Model file for the job. Use its own axes, mm. A direction names the side the tool comes from. Coordinates: 2 decimals unless noted, no trailing zeros. Write each loop counter-clockwise with the first axis right and the second up, starting at its lowest first coordinate (ties: lowest second). Pieces come first, ordered by that corner, then holes. Notation, with made-up numbers: M 25.25,-27.75 L 58.25,-27.75 A22 ccw 58.25,4.25 Z; hole C -3,40 d5. An arc over 180 degrees is marked long. Use CSV: the item, a comma, the result in double quotes. Start each with the question number.
from build123d import *

# Parameters (mm, degrees)
SKETCH1_W                        = 70
SKETCH1_H                        = 100
SKETCH1_W_2                      = 58
SKETCH1_H_2                      = 88
MAIN_BODY_DEPTH                  = 50
BACK_WIRE_HOLE_REACH             = 102
SKETCH3_R                        = 1.5
FRONT_WIRE_HOLE_REACH            = 102
SKETCH6_R                        = 1.5
SKETCH4_W                        = 70
SKETCH4_H                        = 6
BACK_LIP_DEPTH                   = 10
SKETCH5_R                        = 1.5
BACK_LIP_HOLES_DEPTH             = 35
SKETCH2_R                        = 1.5
GEARED_ARM_HOLE_DEPTH            = 6
SKETCH10_W                       = 23
SKETCH10_H                       = 8.7393957
SERVO_MOUNT_MAIN_EXTRUSION_DEPTH = 58
WING_CONNECTION_SLOT_DEPTH       = 6


with BuildPart() as part:
    # Sketch1 → main_body (new body)
    with BuildSketch(Plane(origin=(0, 0, 0), x_dir=(1, 0, 0), z_dir=(0, 1, 0))):
        with Locations((0, -1.59009009)):
            Rectangle(SKETCH1_W, SKETCH1_H)
        with Locations((0, -1.59009009)):
            Rectangle(SKETCH1_W_2, SKETCH1_H_2, mode=Mode.SUBTRACT)
    extrude(amount=MAIN_BODY_DEPTH)

    # Sketch3 → back_wire_hole (cut, up to next)
    with BuildSketch(Plane.XY.offset(51.59009009), mode=Mode.PRIVATE) as back_wire_hole_sk1:
        with Locations((0, 25)):
            Circle(SKETCH3_R)
    back_wire_hole_tool1 = extrude(back_wire_hole_sk1.sketch, amount=-BACK_WIRE_HOLE_REACH, mode=Mode.PRIVATE) & part.part
    add(back_wire_hole_tool1.solids().sort_by_distance((0, 25, 51.59009))[0], mode=Mode.SUBTRACT)

    # Sketch6 → front_wire_hole (cut, up to next)
    with BuildSketch(Plane(origin=(0, 0, -48.40990991), x_dir=(-1, 0, 0), z_dir=(0, 0, -1)), mode=Mode.PRIVATE) as front_wire_hole_sk1:
        with Locations((0, 25)):
            Circle(SKETCH6_R)
    front_wire_hole_tool1 = extrude(front_wire_hole_sk1.sketch, amount=-FRONT_WIRE_HOLE_REACH, mode=Mode.PRIVATE) & part.part
    add(front_wire_hole_tool1.solids().sort_by_distance((0, 25, -48.40991))[0], mode=Mode.SUBTRACT)

    # Sketch4 → back_lip (add)
    with BuildSketch(Plane.XY.offset(51.59009009)):
        with Locations((0, 31)):
            Rectangle(SKETCH4_W, SKETCH4_H)
    back_lip = extrude(amount=BACK_LIP_DEPTH)

    # back_lip_mirror: back_lip across plane
    add(back_lip.mirror(Plane.ZX.offset(25)))

    # Sketch5 → back_lip_holes (cut, through all)
    with BuildSketch(Plane(origin=(0, 34, 0), x_dir=(1, 0, 0), z_dir=(0, 1, 0))):
        with Locations((4, -55.59009009)):
            Circle(SKETCH5_R)
        with Locations((30, -55.59009009)):
            Circle(SKETCH5_R)
        with Locations((-30, -55.59009009)):
            Circle(SKETCH5_R)
        with Locations((-4, -55.59009009)):
            Circle(SKETCH5_R)
    extrude(amount=-BACK_LIP_HOLES_DEPTH, mode=Mode.SUBTRACT)

    # Sketch2 → geared_arm_hole (cut)
    with BuildSketch(Plane(origin=(35, 0, 0), x_dir=(0, 0, -1), z_dir=(1, 0, 0))):
        with Locations((-1.59009009, 25)):
            Circle(SKETCH2_R)
    geared_arm_hole = extrude(amount=-GEARED_ARM_HOLE_DEPTH, mode=Mode.SUBTRACT)

    # geared_arm_hole_mirror: geared_arm_hole across plane
    add(geared_arm_hole.mirror(Plane(origin=(0, 0, 0), x_dir=(0, 0, 1), z_dir=(1, 0, 0))), mode=Mode.SUBTRACT)

    # Sketch10 → servo_mount_main_extrusion (add)
    with BuildSketch(Plane(origin=(-29, 0, 0), x_dir=(0, 0, -1), z_dir=(1, 0, 0))):
        with Locations((32.100688533, 4.36969785)):
            Rectangle(SKETCH10_W, SKETCH10_H)
        with Locations((32.100688533, 45.63030215)):
            Rectangle(SKETCH10_W, SKETCH10_H)
    extrude(amount=SERVO_MOUNT_MAIN_EXTRUSION_DEPTH)

    # Sketch11 → wing_connection_slot (cut)
    with BuildSketch(Plane(origin=(35, 0, 0), x_dir=(0, 0, -1), z_dir=(1, 0, 0))):
        with BuildLine():
            ThreePointArc((-32.317240778, 42.63125), (-33.09009009, 25), (-32.317240778, 7.36875))
            ThreePointArc((-32.317240778, 7.36875), (-30.691743999, 6.005753221), (-29.32874722, 7.63125))
            ThreePointArc((-29.32874722, 7.63125), (-30.09009009, 25), (-29.32874722, 42.36875))
            ThreePointArc((-29.32874722, 42.36875), (-30.691743999, 43.994246779), (-32.317240778, 42.63125))
        make_face()
    wing_connection_slot = extrude(amount=-WING_CONNECTION_SLOT_DEPTH, mode=Mode.SUBTRACT)

    # wing_connection_slot_mirror: wing_connection_slot across plane
    add(wing_connection_slot.mirror(Plane(origin=(0, 0, 0), x_dir=(0, 0, 1), z_dir=(1, 0, 0))), mode=Mode.SUBTRACT)


solid = part.part
1) Two-plate mould, pull along X, no slides. Class faces 1 (the face through (0, 8, 51.59)), 2 (the face through (28.89, 19.04, 54.58)), 3 (the face through (0, 4, -20.601)): pulls with the +X half, pulls with the -X half, needs draft (parallel to the pull), parting line crosses it, or undercut.
2) Band-saw the part on C-C on x = -14. List the corners of the cut face in (y, z), then the cut area to 3 significant figures.
3) Band-saw the part on A-A on x = 4. List the corners of the cut face in (y, z), then the cut area to 3 significant figures.
4) Tool access for faces 4 (the face through (0, 41.261, -31)), 5 (the face through (-32.04, 24.76, 30.09)), 6 (the face through (0, 42, 51.59)), 7 (the face through (0, 27, 51.59)): list every direction of +Z, -Z, +X, -X, +Y, -Y with a clear straight run to the whole face (end or side of a thin tool).
5) Drop flat-ended pins along their axis: P1, Ø13, axis at x = -14.5, y = 7, coming from the +Z side; P2, Ø11, axis at x = 5.5, z = 57.5, coming from the +Y side; P3, Ø5, axis at x = -8, z = 57, coming from the -Y side. Give the stop position or say it passes through.
6) Wall check: L1, parallel to Z at x = -12, y = 16.5; L2, parallel to X at y = 25, z = 28.5; L3, parallel to Y at x = 18, z = -33. Give the ranges that are in metal, low to high. Write a range as [from, to].
7) Band-saw the part on B-B on z = 15. List the corners of the cut face in (x, y).
8) Band-saw the part on D-D on z = -40. List the corners of the cut face in (x, y), then the cut area to 3 significant figures.
Findings below:
1,face 1,"needs draft"
1,face 2,"undercut"
1,face 3,"undercut"
2,outline,"M 0,-48.41 L 50,-48.41 L 50,-20.6 L 41.26,-20.6 L 41.26,-42.41 L 8.74,-42.41 L 8.74,-20.6 L 0,-20.6 Z; M 0,45.59 L 50,45.59 L 50,51.59 L 34,51.59 L 34,61.59 L 28,61.59 L 28,51.59 L 22,51.59 L 22,61.59 L 16,61.59 L 16,51.59 L 0,51.59 Z"
2,area,"1,100 mm2"
3,outline,"M 0,-48.41 L 50,-48.41 L 50,-20.6 L 41.26,-20.6 L 41.26,-42.41 L 8.74,-42.41 L 8.74,-20.6 L 0,-20.6 Z; M 0,45.59 L 50,45.59 L 50,51.59 L 34,51.59 L 34,54.09 L 28,54.09 L 28,51.59 L 22,51.59 L 22,54.09 L 16,54.09 L 16,51.59 L 0,51.59 Z; M 16,57.09 L 22,57.09 L 22,61.59 L 16,61.59 Z; M 28,57.09 L 34,57.09 L 34,61.59 L 28,61.59 Z"
3,area,"1,070 mm2"
4,face 4,"none"
4,face 5,"+X, -X"
4,face 6,"+Z, +X, -X, +Y"
4,face 7,"+Z, +X, -X"
5,P1,"stops at z = 51.59"
5,P2,"stops at y = 34"
5,P3,"stops at y = 16"
6,L1,"z = [-48.41, -42.41], [45.59, 61.59]"
6,L2,"x = [-35, -29], [29, 35]"
6,L3,"y = [0, 8.74], [41.26, 50]"
7,outline,"M -35,0 L -29,0 L -29,50 L -35,50 Z; M 29,0 L 35,0 L 35,50 L 29,50 Z"
8,outline,"M -35,0 L 35,0 L 35,50 L -35,50 Z; hole M -29,8.74 L 29,8.74 L 29,41.26 L -29,41.26 Z"
8,area,"1,610 mm2"
